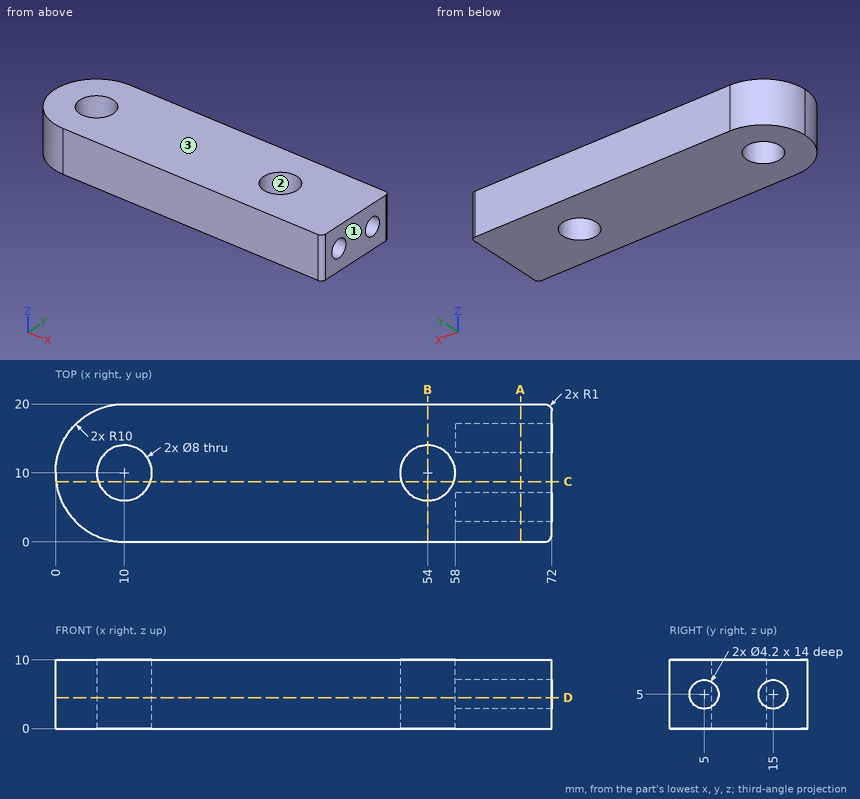
Design review of the part shown in the three views and the two pictorial views. Dimensions are in mm from the part's minimum x, y and z. Round coordinates to 2 decimals unless told otherwise and drop trailing zeros. Write each loop counter-clockwise with the first axis right and the second up, starting at its lowest first coordinate (ties: lowest second). Pieces come first, ordered by that corner, then holes. Notation, with made-up numbers: (-34.5, 53) - (-5.5, 53) arc R28 ccw to (-5.5, 83) - close; hole circle Ø11 at (-4.5, -11). An arc over 180 degrees is marked (long way). Write item = value, one per line. Start each with the question number.
1. Wall thickness on L1, parallel to Y at x = 64, z = 5; L2, parallel to Y at x = 10, z = 4; L3, parallel to X at y = 10.25, z = 6.75: over which ranges is each line inside the solid? List them lowest first.
2. Consider section A-A on x = 67.5. State the section outline as (y, z) points.
3. Consider section C-C on y = 8.75. State the section outline as (x, z) points, plus the area to 3 significant figures.
4. Consider section D-D on z = 4.5. Give the number of separate pieces and of enclosed holes in the cut face, plus the area to 3 significant figures.
5. Consider section B-B on x = 54. State the section outline as (y, z) points.
6. For pin 1 Ø1.5 at (y, z) = (10.5, 3.5) entering from -X; pin 2 Ø3.5 at (y, z) = (15, 5) entering from -X; pin 3 Ø5 at (x, y) = (10, 10) entering from -Z; pin 4 Ø1 at (y, z) = (6, 4.5) entering from -X, all flat-tipped, find the tip position at first contact; note any pin that passes through.
7. Draft analysis for pull direction X (two halves, no side actions). For the marked faces 1, 2 and 3, state which applies: released by +X, released by -X, zero draft, split by the parting line, or undercut.
Evaluation:
q1.L1 = 0 to 2.9, 7.1 to 12.9, 17.1 to 20
q1.L2 = 0 to 6, 14 to 20
q1.L3 = 0 to 6.01, 13.99 to 50.01, 57.99 to 72
q2.outline = (0, 0) - (20, 0) - (20, 10) - (0, 10) - close; hole circle Ø4.2 at (5, 5); hole circle Ø4.2 at (15, 5)
q3.outline = (0.08, 0) - (6.2, 0) - (6.2, 10) - (0.08, 10) - close; (13.8, 0) - (50.2, 0) - (50.2, 10) - (13.8, 10) - close; (57.8, 0) - (72, 0) - (72, 10) - (57.8, 10) - close
q3.area = 567 mm2
q4.separate_pieces = 1
q4.enclosed_holes = 2
q4.area = 1,180 mm2
q5.outline = (0, 0) - (6, 0) - (6, 10) - (0, 10) - close; (14, 0) - (20, 0) - (20, 10) - (14, 10) - close
q6.pin_1 = 0
q6.pin_2 = 0.54
q6.pin_3 = through
q6.pin_4 = 0.63
q7.face_1 = released by +X
q7.face_2 = undercut
q7.face_3 = zero draft
